Can you work these out from the model? Positions are in its coordinate system, mm. Face numbers are marked on the shaded views. A direction names the side the tool comes from. Coordinates: 2 decimals unless noted, no trailing zeros. Order: outer loops, then holes, each group sorted by start corner. A loop starts at its lowest first (then second) coordinate and runs counter-clockwise, first axis right, second up. Notation, with made-up numbers: (37, 53) -> (89, 53) arc R18 ccw to (89, 72) -> close; hole circle Ø7 at (25, 6). An arc over 180 degrees is marked (long way). Answer in a Markdown table with one row per item.
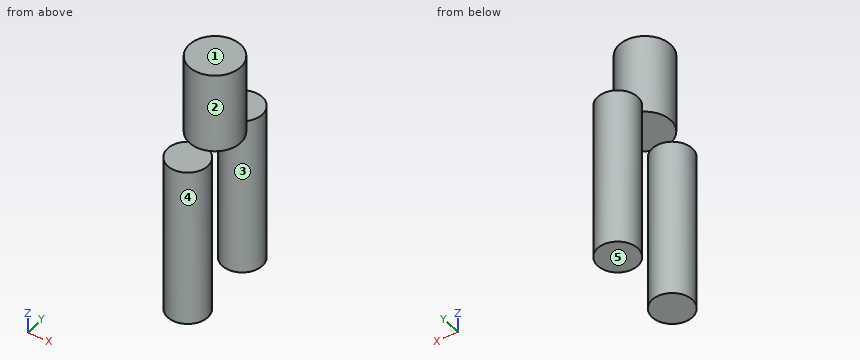
```python
from build123d import *

# Parameters (mm, degrees)
SKETCH1_R             = 1.5875
BOSS_EXTRUDE1_DEPTH   = 12.7
BOSS_EXTRUDE1_2_DEPTH = 12.7
SKETCH2_R             = 2.032
BOSS_EXTRUDE2_DEPTH   = 6.35


with BuildPart() as part:
    # Sketch1 → Boss-Extrude1 (new body)
    with BuildSketch(Plane.XY):
        with Locations((0, 12.7)):
            Circle(SKETCH1_R)
    extrude(amount=-BOSS_EXTRUDE1_DEPTH)



with BuildPart() as body_2:
    # Sketch1 → Boss-Extrude1 2 (new body)
    with BuildSketch(Plane.XY):
        with Locations((0, 19.05)):
            Circle(SKETCH1_R)
    extrude(amount=-BOSS_EXTRUDE1_2_DEPTH)


with BuildPart() as part_1:
    add(part.part)

    add(body_2.part)  # Boss-Extrude2 merges body 2
    # Sketch2 → Boss-Extrude2 (add)
    with BuildSketch(Plane.XY):
        with Locations(Location((0, 15.875, 0), (0, 0, 115.050153991))):
            Circle(SKETCH2_R)
    extrude(amount=BOSS_EXTRUDE2_DEPTH)


solid = part_1.part
```
(1) Suppose I cut it at D-D (y = 11.75). Please give me the cut outline in (x, z).
Response values:
| item | result |
|---|---|
| outline | (-1.27, -12.7) -> (1.27, -12.7) -> (1.27, 0) -> (-1.27, 0) -> close |
(2) On a 3-axis mill with a long thin cutter (end or side, diameter ignored), from which of +Z, -Z, +X, -X, +Y, -Y can I reach the whole of each face in a straight line? I mean the marked faces 4 and 5. Say none if no direction works.
Response values:
| item | result |
|---|---|
| face 4 | -Z |
| face 5 | -Z, +X, -X, +Y, -Y |
(3) Will this pin go through, and if not, where does the flat tip stop? pin 1 Ø0.9 at (x, y) = (-0.5, 13) entering from +Z.
Response values:
| item | result |
|---|---|
| pin 1 | z = 0 |
(4) Suppose I cut it at C-C (y = 19.05). Please give me the cut outline in (x, z), and give its area (3 significant figures).
Response values:
| item | result |
|---|---|
| outline | (-1.59, -12.7) -> (1.59, -12.7) -> (1.59, 0) -> (-1.59, 0) -> close |
| area | 40.3 mm2 |
(5) Suppose I cut it at B-B (x = 0). Please give me the cut outline in (y, z), and give its area (3 significant figures).
Response values:
| item | result |
|---|---|
| outline | (11.11, -12.7) -> (14.29, -12.7) -> (14.29, 0) -> (17.46, 0) -> (17.46, -12.7) -> (20.64, -12.7) -> (20.64, 0) -> (17.91, 0) -> (17.91, 6.35) -> (13.84, 6.35) -> (13.84, 0) -> (11.11, 0) -> close |
| area | 106 mm2 |
(6) I need wall thicknesses on line 1 (Y direction, x = -0.1, z = -6); line 2 (Z direction, x = -0.4, y = 12); line 3 (Z direction, x = 0.5, y = 15.25). Which ranges of each line are inside material? Lowest first, please. Write a range as [from, to].
Response values:
| item | result |
|---|---|
| line 1 | [11.12, 14.28], [17.47, 20.63] |
| line 2 | [-12.7, 0] |
| line 3 | [0, 6.35] |
(7) We'd pull the mould along Y, two halves only. Please class the marked faces 1, 2 and 3: +Y half, -Y half, draft (parallel to the pull), parting line (faces both ways), or undercut.
Response values:
| item | result |
|---|---|
| face 1 | draft |
| face 2 | parting line |
| face 3 | undercut |
